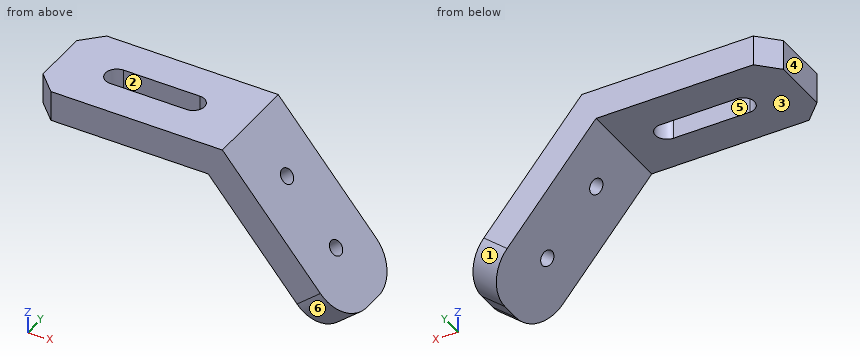
from build123d import *

# Parameters (mm, degrees)
F1_DEPTH = 12.5
F3_DEPTH = 43.4455230334
F5_D     = 4
F6_R     = 10
F7_SIZE  = 5


with BuildPart() as f1:
    # F0 (on Front) → F1 (new body, symmetric)
    with BuildSketch(Plane.XZ):
        Polygon((0, 8), (0, 0), (46.2695387348, 0), (76.0110249394, -35.4445230334), (82.1393804843, -30.3022221559), (50, 8), align=None)
    extrude(amount=F1_DEPTH, both=True)

    # F2 (on face) → F3 (cut, through all)
    with BuildSketch(Plane.XY.offset(8)):
        with BuildLine():
            ThreePointArc((15, 3), (12, 0), (15, -3))
            Line((15, -3), (35, -3))
            ThreePointArc((35, -3), (38, 0), (35, 3))
            Line((35, 3), (15, 3))
        make_face()
    extrude(amount=-F3_DEPTH, mode=Mode.SUBTRACT)

    # F5 (through all)
    with Locations(Plane(origin=(33.2804354537, 0, 27.9256011146), x_dir=(0, 1, 0), z_dir=(0.7660444431, 0, 0.6427876097))):
        with Locations((0, -41.0110249394), (0, -61.0110249394)):
            Hole(F5_D / 2)

    # F6
    f6_edges = [f1.edges().sort_by_distance(p)[0] for p in [
        (79.075203, -12.5, -32.873373),
        (79.075203, 12.5, -32.873373),
    ]]
    fillet(f6_edges, radius=F6_R)

    # F7
    f7_edges = [f1.edges().sort_by_distance(p)[0] for p in [
        (0, -12.5, 4),
        (0, 12.5, 4),
    ]]
    chamfer(f7_edges, length=F7_SIZE)


solid = f1.part
Model file for the job. Use its own axes, mm. Face numbers are marked on the shaded views. A direction names the side the tool comes from. Round coordinates to 2 decimals unless told otherwise and drop trailing zeros. Loops run counter-clockwise (first coordinate to the right, second up) from the corner with the lowest first, then second, coordinate; pieces in that order, holes last. Notation, with made-up numbers: (79.25, -36) -> (117.25, -36) arc R13 ccw to (117.25, -11) -> close; hole circle Ø11 at (-22.5, 6). An arc over 180 degrees is marked (long way). Answer as CSV lines item,"result". Start each with the question number.
1) Pin check, flat tips, straight feed: P1, Ø6, axis at y = 6.5, z = -25.5, coming from the -X side; P2, Ø5, axis at x = 62.5, y = -1.5, coming from the -Z side; P3, Ø3, axis at y = -5.5, z = -4.5, coming from the -X side. Stop position of each tip, or through.
2) Mould opens along X. For the marked faces 4, 5 and 6 say: +X half, -X half, draft (parallel to the pull), parting line (faces both ways), or undercut.
3) Slice it at A-A (y = 0). List the corners of the cut face in (x, z).
4) Probe line 1 along Z through (x, y) = (14, 6.5); line 2 along Z through (x, y) = (70.5, -1); line 3 along Y through (x, z) = (57, -3.5). List the from-to ranges inside material, lowest first.
5) Tool access for the marked faces 1, 2 and 3: list every direction of +Z, -Z, +X, -X, +Y, -Y with a clear straight run to the whole face (end or side of a thin tool).
Filled in:
1,P1,"stops at x = 65.15"
1,P2,"stops at z = -22.32"
1,P3,"stops at x = 48.79"
2,face 4,"-X half"
2,face 5,"undercut"
2,face 6,"+X half"
3,outline,"(0, 0) -> (12, 0) -> (12, 8) -> (0, 8) -> close; (38, 0) -> (46.27, 0) -> (52.23, -7.1) -> (58.36, -1.96) -> (50, 8) -> (38, 8) -> close; (54.8, -10.17) -> (65.08, -22.42) -> (71.21, -17.28) -> (60.93, -5.02) -> close; (67.65, -25.49) -> (76.01, -35.44) -> (82.14, -30.3) -> (73.78, -20.34) -> close"
4,line 1,"z = 0 to 8"
4,line 2,"z = -28.88 to -22.75, -18.23 to -16.43"
4,line 3,"y = -12.5 to -1.07, 1.07 to 12.5"
5,face 1,"-Z, +X, +Y"
5,face 2,"+Z, -Z"
5,face 3,"-Z, -X, +Y, -Y"
